from build123d import *

# Parameters (mm, degrees)
ESQUISSE1_W        = 8
ESQUISSE1_H        = 8
BOSS_EXTRU_1_DEPTH = 3
CHANFREIN1_SIZE    = 1
ESQUISSE2_W        = 5
ESQUISSE2_H        = 5
BOSS_EXTRU_2_DEPTH = 2


with BuildPart() as part:
    # Esquisse1 → Boss.-Extru.1 (new body)
    with BuildSketch(Plane(origin=(0, 0, 0), x_dir=(1, 0, 0), z_dir=(0, 1, 0))):
        Rectangle(ESQUISSE1_W, ESQUISSE1_H)
    extrude(amount=BOSS_EXTRU_1_DEPTH)

    # Chanfrein1
    chanfrein1_edges = [part.edges().sort_by_distance(p)[0] for p in [
        (0, 0, 4),
        (-4, 0, 0),
        (0, 0, -4),
        (4, 0, 0),
    ]]
    chamfer(chanfrein1_edges, length=CHANFREIN1_SIZE)

    # Esquisse2 → Boss.-Extru.2 (add)
    with BuildSketch(Plane(origin=(0, 3, 0), x_dir=(1, 0, 0), z_dir=(0, 1, 0))):
        Rectangle(ESQUISSE2_W, ESQUISSE2_H)
    extrude(amount=BOSS_EXTRU_2_DEPTH)


solid = part.part
The listing builds one solid part. Answer for the finished solid, in the listing's coordinates (mm). A direction names the side the tool comes from. Give positions to 0.01 mm unless a question says otherwise; leave off trailing zeros. Write each loop counter-clockwise with the first axis right and the second up, starting at its lowest first coordinate (ties: lowest second). Pieces come first, ordered by that corner, then holes. Notation, with made-up numbers: (79, 65.5) -> (108, 65.5) arc R18 cw to (108, 92.5) -> close; hole circle Ø4 at (-8.5, 84). An arc over 180 degrees is marked (long way). One line per question, with ' | ' between items. Start each with the question number.
1. Section A-A (x = 0.25) is taken. Determine the outline of the cut face in (y, z), plus the area to 3 significant figures.
2. Given pin 1 Ø2 at (x, y) = (0.5, 4.5) entering from +Z; pin 2 Ø2 at (x, y) = (0, 4.5) entering from -Z; pin 3 Ø1 at (x, z) = (0, 0) entering from -Y; pin 4 Ø1 at (y, z) = (4, -1) entering from +X, each flat-ended and moving along its own axis, determine where each tip first touches the part or whether it passes through.
3. Section D-D (x = 3.25) is taken. Determine the outline of the cut face in (y, z).
4. Section B-B (z = 1) is taken. Determine the outline of the cut face in (x, y).
5. For faces 1 (the flat face through (0, 4, 2.5)), 2 (the flat face through (0, 4, -2.5)), 3 (the flat face through (-2.5, 4, 0)), 4 (the flat face through (2.5, 4, 0)), 5 (the flat face through (-0.1, 0.5, 3.5)), determine the directions among +Z, -Z, +X, -X, +Y, -Y from which every point of the face is accessible in a straight line to the end or side of a thin tool.
6. Section C-C (y = 0.4) is taken. Determine the outline of the cut face in (x, z).
7. Find the intervals of material crossed by probe 1 along Z at (x, y) = (2, 4.35); probe 2 along Y at (x, z) = (-1.75, 2.75), in increasing order.
Response values:
1) outline: (0, -3) -> (1, -4) -> (3, -4) -> (3, -2.5) -> (5, -2.5) -> (5, 2.5) -> (3, 2.5) -> (3, 4) -> (1, 4) -> (0, 3) -> close | area: 33.0 mm2
2) pin 1: z = 2.5 | pin 2: z = -2.5 | pin 3: y = 0 | pin 4: x = 2.5
3) outline: (0.25, -3.25) -> (1, -4) -> (3, -4) -> (3, 4) -> (1, 4) -> (0.25, 3.25) -> close
4) outline: (-4, 1) -> (-3, 0) -> (3, 0) -> (4, 1) -> (4, 3) -> (2.5, 3) -> (2.5, 5) -> (-2.5, 5) -> (-2.5, 3) -> (-4, 3) -> close
5) face 1: +Z, +X, -X, +Y | face 2: -Z, +X, -X, +Y | face 3: +Z, -Z, -X, +Y | face 4: +Z, -Z, +X, +Y | face 5: +Z, +X, -X, -Y
6) outline: (-3.4, -3.4) -> (3.4, -3.4) -> (3.4, 3.4) -> (-3.4, 3.4) -> close
7) probe 1: -2.5 to 2.5 | probe 2: 0 to 3
